Here's how the part is built. I have some questions about the finished solid (model axes, mm). Face numbers are marked on the shaded views. Round coordinates to 2 decimals unless told otherwise and drop trailing zeros. Order: outer loops, then holes, each group sorted by start corner. A loop starts at its lowest first (then second) coordinate and runs counter-clockwise, first axis right, second up. Notation, with made-up numbers: (-34.75, 54.25) -> (8.25, 54.25) arc R18 ccw to (8.25, 66.25) -> close; hole circle Ø8 at (-17, -39.75). An arc over 180 degrees is marked (long way). Answer in a Markdown table with one row per item.
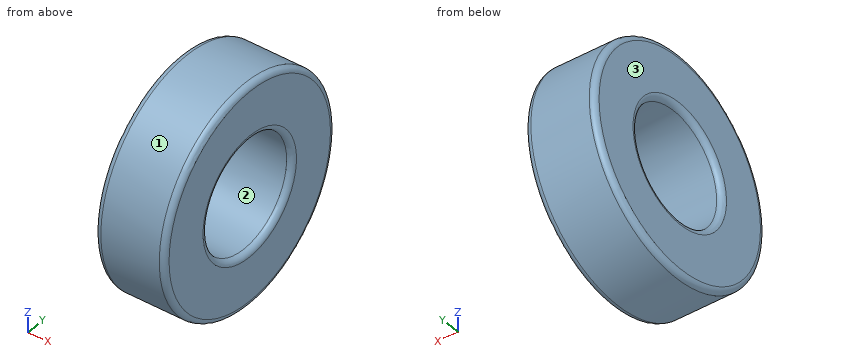
```python
from build123d import *

# Parameters (mm, degrees)
CROQUIS1_R              = 8
CROQUIS1_R_2            = 4
SALIENTE_EXTRUIR1_DEPTH = 5
REDONDEO1_R             = 0.4


with BuildPart() as part:
    # Croquis1 → Saliente-Extruir1 (new body)
    with BuildSketch(Plane(origin=(0, 0, 0), x_dir=(0, 0, -1), z_dir=(1, 0, 0))):
        Circle(CROQUIS1_R)
        Circle(CROQUIS1_R_2, mode=Mode.SUBTRACT)
    extrude(amount=SALIENTE_EXTRUIR1_DEPTH)

    # Redondeo1
    redondeo1_edges = [part.edges().sort_by_distance(p)[0] for p in [
        (0, 0, 8),
        (5, 0, 8),
        (0, 0, 4),
        (5, 0, 4),
    ]]
    fillet(redondeo1_edges, radius=REDONDEO1_R)


solid = part.part
```
1. Please list where these lines run through material, in increasing order: line 1 along Y through (x, z) = (2.4, 0); line 2 along Y through (x, z) = (3.5, -3); line 3 along Z through (x, y) = (4.1, 2.25).
Numbers:
| item | result |
|---|---|
| line 1 | y = -8 to -4, 4 to 8 |
| line 2 | y = -7.42 to -2.65, 2.65 to 7.42 |
| line 3 | z = -7.68 to -3.31, 3.31 to 7.68 |
2. Suppose I cut it at C-C on x = 3.95. Write out the boundary of the cut face in (y, z).
Numbers:
| item | result |
|---|---|
| outline | circle Ø16 at (0, 0); hole circle Ø8 at (0, 0) |
3. Suppose I cut it at A-A on y = 0. Write out the boundary of the cut face in (x, z).
Numbers:
| item | result |
|---|---|
| outline | (0, -7.6) arc R0.4 ccw to (0.4, -8) -> (4.6, -8) arc R0.4 ccw to (5, -7.6) -> (5, -4.4) arc R0.4 ccw to (4.6, -4) -> (0.4, -4) arc R0.4 ccw to (0, -4.4) -> close; (0, 4.4) arc R0.4 ccw to (0.4, 4) -> (4.6, 4) arc R0.4 ccw to (5, 4.4) -> (5, 7.6) arc R0.4 ccw to (4.6, 8) -> (0.4, 8) arc R0.4 ccw to (0, 7.6) -> close |
4. We'd pull the mould along Y, two halves only. Please class the marked faces 1, 2 and 3: released by +Y, released by -Y, zero draft, split by the parting line, or undercut.
Numbers:
| item | result |
|---|---|
| face 1 | split by the parting line |
| face 2 | undercut |
| face 3 | zero draft |
5. For pin 1 Ø2 at (x, y) = (2, -4.5) entering from -Z; pin 2 Ø2 at (x, y) = (1.5, 6.5) entering from -Z, each with a flat end and sliding along its axis, tell me the tip position at first contact or that it passes through.
Numbers:
| item | result |
|---|---|
| pin 1 | stops at z = -7.19 |
| pin 2 | stops at z = -5.81 |
